The listing builds one solid part. Answer for the finished solid, in the listing's coordinates (mm). Face numbers are marked on the shaded views. A direction names the side the tool comes from. Round coordinates to 2 decimals unless told otherwise and drop trailing zeros. Loops run counter-clockwise (first coordinate to the right, second up) from the corner with the lowest first, then second, coordinate; pieces in that order, holes last. Notation, with made-up numbers: M 17.5,12 L 57.5,12 A23 cw 57.5,45 Z; hole C -33,-4 d3. An arc over 180 degrees is marked long. Answer as a JSON object with one key per item and string values.
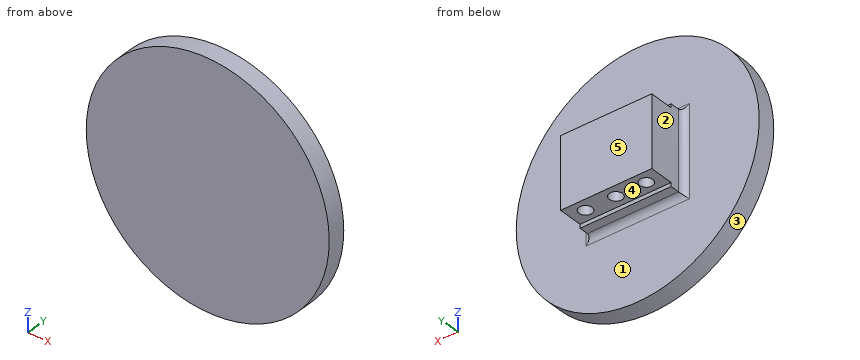
Autodesk Inventor part; units mm, degrees
ref_plane "YZ Plane" through (0, 0, 0) normal (1, 0, 0) x (0, 1, 0)
ref_plane "XZ Plane" through (0, 0, 0) normal (0, 1, 0) x (-1, 0, 0)
ref_plane "XY Plane" through (0, 0, 0) normal (0, 0, 1) x (1, 0, 0)
sketch "Sketch1" plane through (0, 0, 0) normal (0, 1, 0) x (-1, 0, 0)
  line L0 (-15, 11.75) -> (-15, -11.75)
  line L1 (-15, -11.75) -> (15, -11.75)
  line L2 (15, -11.75) -> (15, 11.75)
  line L3 (15, 11.75) -> (-15, 11.75)
  line L4 (-15, 11.75) -> (15, -11.75) construction
  line L5 (-15, -11.75) -> (15, 11.75) construction
  point P0 (0, 0)
  dimension "d0" = 23.5
  dimension "d1" = 30
extrude "Extrusion1" add sketch "Sketch1" along normal blind 8
sketch "Sketch2" plane through (-15, 0, 11.75) normal (0, 0, 1) x (1, 0, 0)
  circle A0 centre (15, 4) radius 1.5
  line L0 (0, 8) -> (30, 8)
  point P0 (15, 0)
  dimension "d4" = 3
  dimension "d5" = 8
  dimension "d6" = 4
hole "Hole1" at (0, 4, 11.75) direction (0, 0, -1) diameter 3.88 depth 7 countersink diameter 4.34 countersink angle 7
pattern_linear "Rectangular Pattern1" count 2 spacing 10 along (1, 0, 0) count 2 spacing 10 along (-1, 0, 0) of "Hole1"
mirror "Mirror1" about plane through (0, 0, 0) normal (0, 0, 1) of "Hole1", "Rectangular Pattern1"
sketch "Sketch3" plane through (0, 0, 0) normal (0, -1, 0) x (1, 0, 0)
  line L0 (-15, -13) -> (-15, 13)
  line L1 (-15, 13) -> (15, 13)
  line L2 (15, 13) -> (15, -13)
  line L3 (15, -13) -> (-15, -13)
  line L4 (-15, -13) -> (15, 13) construction
  line L5 (-15, 13) -> (15, -13) construction
  point P0 (0, 0)
  dimension "d20" = 26
  dimension "d21" = 30
extrude "Extrusion2" add sketch "Sketch3" along normal blind 5
sketch "Sketch4" plane through (0, -5, 0) normal (0, -1, 0) x (1, 0, 0)
  circle A0 centre (0, 0) radius 40
  dimension "d24" = 80
extrude "Extrusion3" add sketch "Sketch4" along normal blind 6
fillet "Fillet1" radius 2 4 edges at (0, -5, 13) (15, -5, 0) (0, -5, -13) (-15, -5, 0)
properties part number "cycloid_fixing_base"
Item 1: Which of the six approach directions +Z, -Z, +X, -X, +Y, -Y give full straight-line access (tool end or side, diameter ignored) to the marked faces 1, 2, 3, 4 and 5?
Values follow:
{"face 1": "+Y", "face 2": "+Z, -Z, -X, +Y", "face 3": "+Y, -Y", "face 4": "-Z, +X, -X, +Y", "face 5": "+Z, -Z, +X, -X, +Y"}
Item 2: Straight lines are drawn through the part: line 1 (X direction, y = 4, z = 6.25); line 2 (Y direction, x = -10, z = -6); line 3 (Y direction, x = -17, z = 31.5). For each, find the intervals that lie inside material, in ascending order.
Values follow:
{"line 1": "-15 to -11.94, -8.06 to -1.94, 1.94 to 8.06, 11.94 to 15", "line 2": "-11 to 2.06, 5.94 to 8", "line 3": "-11 to -5"}
Item 3: Flat-ended cylindrical pins translate along their axes: P1, Ø2, axis at y = 5.5, z = 11, coming from the -X side; P2, Ø5, axis at x = 10, y = 4, coming from the -Z side; P3, Ø3, axis at x = -16, y = 1.5, coming from the +Z side. Find the tip coordinate at first contact, or state that the pin passes through.
Values follow:
{"P1": "x = -15", "P2": "z = -11.75", "P3": "z = 11.75"}
Item 4: The part is cut by section C-C (y = -6). Give the vertices of the cut face in (x, z).
Values follow:
{"outline": "C 0,0 d80"}
Item 5: The part is cut by section D-D (z = -27). Give the vertices of the cut face in (x, y), then the cut area to 3 significant figures.
Values follow:
{"outline": "M -29.51,-11 L 29.51,-11 L 29.51,-5 L -29.51,-5 Z", "area": "354 mm^2"}
Item 6: The part is cut by section A-A (z = 0). Give the vertices of the cut face in (x, y), then the cut area to 3 significant figures.
Values follow:
{"outline": "M -40,-11 L 40,-11 L 40,-5 L 17,-5 A2 cw 15,-3 L 15,8 L -15,8 L -15,-3 A2 cw -17,-5 L -40,-5 Z", "area": "872 mm^2"}
Item 7: The part is cut by section B-B (x = 10). Give the vertices of the cut face in (y, z), then the cut area to 3 significant figures.
Values follow:
{"outline": "M -11,-38.73 L -5,-38.73 L -5,-15 A2 cw -3,-13 L 0,-13 L 0,-11.75 L 1.83,-11.75 L 2.06,-7.99 L 2.06,-4.75 L 5.94,-4.75 L 5.94,-7.99 L 6.17,-11.75 L 8,-11.75 L 8,11.75 L 6.17,11.75 L 5.94,7.99 L 5.94,4.75 L 2.06,4.75 L 2.06,7.99 L 1.83,11.75 L 0,11.75 L 0,13 L -3,13 A2 cw -5,15 L -5,38.73 L -11,38.73 Z", "area": "728 mm^2"}
